Geometry: final body of the model. Coordinates: model frame, mm. Face numbers are marked on the shaded views. A direction names the side the tool comes from. Round coordinates to 2 decimals unless told otherwise and drop trailing zeros. Loops run counter-clockwise (first coordinate to the right, second up) from the corner with the lowest first, then second, coordinate; pieces in that order, holes last. Notation, with made-up numbers: (51, -18.75) - (67, -18.75) arc R19 cw to (67, 10.25) - close; hole circle Ø6 at (-22.75, 20). An arc over 180 degrees is marked (long way). Use CSV: the item, a comma, the result in double quotes.
from build123d import *

# Parameters (mm, degrees)
F1_DEPTH = 2
F3_DEPTH = 15
F4_R     = 3


with BuildPart() as f1:
    # F0 (on Top) → F1 (new body)
    with BuildSketch(Plane.XY):
        with BuildLine():
            ThreePointArc((46.9791666667, 17.11601295), (49.2390004637, 8.6902723394), (50, 0))
            ThreePointArc((50, 0), (49.2390004637, -8.6902723394), (46.9791666667, -17.11601295))
            ThreePointArc((46.9791666667, -17.11601295), (52.0440237461, -31.7330315504), (60, -45))
            ThreePointArc((60, -45), (67.9559762539, -31.7330315504), (73.0208333333, -17.11601295))
            ThreePointArc((73.0208333333, -17.11601295), (70, 0), (73.0208333333, 17.11601295))
            ThreePointArc((73.0208333333, 17.11601295), (67.9559762539, 31.7330315504), (60, 45))
            ThreePointArc((60, 45), (52.0440237461, 31.7330315504), (46.9791666667, 17.11601295))
        make_face()
        with BuildLine():
            ThreePointArc((46.9791666667, -17.11601295), (-50, 0), (46.9791666667, 17.11601295))
            ThreePointArc((46.9791666667, 17.11601295), (52.0440237461, 31.7330315504), (60, 45))
            ThreePointArc((60, 45), (-75, 0), (60, -45))
            ThreePointArc((60, -45), (52.0440237461, -31.7330315504), (46.9791666667, -17.11601295))
        make_face()
        with BuildLine():
            ThreePointArc((195, 0), (143.7170824513, 71.1512473538), (60, 45))
            ThreePointArc((60, 45), (67.9559762539, 31.7330315504), (73.0208333333, 17.11601295))
            ThreePointArc((73.0208333333, 17.11601295), (128.6902723394, 49.2390004637), (170, 0))
            ThreePointArc((170, 0), (128.6902723394, -49.2390004637), (73.0208333333, -17.11601295))
            ThreePointArc((73.0208333333, -17.11601295), (67.9559762539, -31.7330315504), (60, -45))
            ThreePointArc((60, -45), (143.7170824513, -71.1512473538), (195, 0))
        make_face()
        with BuildLine():
            ThreePointArc((46.9791666667, -17.11601295), (49.2390004637, -8.6902723394), (50, 0))
            ThreePointArc((50, 0), (49.2390004637, 8.6902723394), (46.9791666667, 17.11601295))
            ThreePointArc((46.9791666667, 17.11601295), (45, 0), (46.9791666667, -17.11601295))
        make_face()
        with BuildLine():
            ThreePointArc((75, 0), (74.5035653509, 8.6150304701), (73.0208333333, 17.11601295))
            ThreePointArc((73.0208333333, 17.11601295), (70, 0), (73.0208333333, -17.11601295))
            ThreePointArc((73.0208333333, -17.11601295), (74.5035653509, -8.6150304701), (75, 0))
        make_face()
    extrude(amount=F1_DEPTH)

    # F2 (on face) → F3 (join)
    with BuildSketch(Plane.XY.offset(2)):
        with BuildLine():
            ThreePointArc((60, 45), (-75, 0), (60, -45))
            ThreePointArc((60, -45), (195, 0), (60, 45))
        make_face()
        with BuildLine():
            ThreePointArc((60, -43.3128156554), (-74, 0), (60, 43.3128156554))
            ThreePointArc((60, 43.3128156554), (194, 0), (60, -43.3128156554))
        make_face(mode=Mode.SUBTRACT)
        with BuildLine():
            ThreePointArc((48.0208333333, -17.1755514023), (46, 0), (48.0208333333, 17.1755514023))
            ThreePointArc((48.0208333333, 17.1755514023), (-51, 0), (48.0208333333, -17.1755514023))
        make_face()
        with BuildLine():
            ThreePointArc((46.9791666667, -17.11601295), (-50, 0), (46.9791666667, 17.11601295))
            ThreePointArc((46.9791666667, 17.11601295), (45, 0), (46.9791666667, -17.11601295))
        make_face(mode=Mode.SUBTRACT)
        with BuildLine():
            ThreePointArc((71.9791666667, 17.1755514023), (74, 0), (71.9791666667, -17.1755514023))
            ThreePointArc((71.9791666667, -17.1755514023), (171, 0), (71.9791666667, 17.1755514023))
        make_face()
        with BuildLine():
            ThreePointArc((73.0208333333, 17.11601295), (170, 0), (73.0208333333, -17.11601295))
            ThreePointArc((73.0208333333, -17.11601295), (75, 0), (73.0208333333, 17.11601295))
        make_face(mode=Mode.SUBTRACT)
    extrude(amount=F3_DEPTH)

    # F4
    f4_edges = [f1.edges().sort_by_distance(p)[0] for p in [
        (60, 45, 8.5),
        (60, -45, 8.5),
        (60, 43.312816, 9.5),
        (71.979167, -17.175551, 9.5),
        (73.020833, -17.116013, 8.5),
        (73.020833, 17.116013, 8.5),
        (48.020833, 17.175551, 9.5),
        (46.979167, 17.116013, 8.5),
        (46.979167, -17.116013, 8.5),
        (60, -43.312816, 9.5),
        (48.020833, -17.175551, 9.5),
        (71.979167, 17.175551, 9.5),
    ]]
    fillet(f4_edges, radius=F4_R)


solid = f1.part
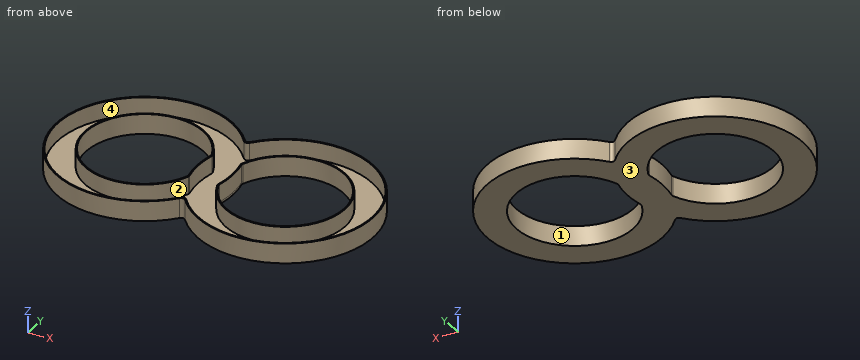
Item 1: Section C-C on z = 13. Give the number of separate pieces and of enclosed holes in the cut face, plus the area to 3 significant figures.
Final values:
separate pieces,"3"
enclosed holes,"3"
area,"1,380 mm²"
Item 2: Pin query (flat end, axial travel): P1, Ø3, axis at y = 26.5, z = 11.5, coming from the -X side; P2, Ø1.5, axis at x = -41.5, z = 5, coming from the -Y side; P3, Ø10, axis at x = -10, z = 7, coming from the -Y side. Return the tip coordinate at first contact, or that it passes through.
Final values:
P1,"stops at x = -70.71"
P2,"stops at y = -62.96"
P3,"stops at y = -74.83"
Item 3: Section B-B on y = 57.5. Return the cut outline in (x, z).
Final values:
outline,"(-48.15, 0) - (48.15, 0) - (48.15, 17) - (46.58, 17) - (46.58, 2) - (-46.58, 2) - (-46.58, 17) - (-48.15, 17) - close; (71.85, 0) - (168.15, 0) - (168.15, 17) - (166.58, 17) - (166.58, 2) - (73.42, 2) - (73.42, 17) - (71.85, 17) - close"
Item 4: Section D-D on y = -30. Return the cut outline in (x, z).
Final values:
outline,"(-68.74, 0) - (-40, 0) - (-40, 17) - (-41.24, 17) - (-41.24, 2) - (-67.65, 2) - (-67.65, 17) - (-68.74, 17) - close; (40, 0) - (80, 0) - (80, 17) - (78.76, 17) - (78.76, 2) - (41.24, 2) - (41.24, 17) - (40, 17) - close; (160, 0) - (188.74, 0) - (188.74, 17) - (187.65, 17) - (187.65, 2) - (161.24, 2) - (161.24, 17) - (160, 17) - close"
Item 5: Reachability of the marked faces 1 and 2 from +Z, -Z, +X, -X, +Y, -Y: full face, straight path, thin tool, end or side. Return the list, or none.
Final values:
face 1,"+Z, -Z"
face 2,"+Z"
Item 6: Section A-A on x = 120. Return the cut outline in (y, z), plus the area to 3 significant figures.
Final values:
outline,"(-75, 0) - (-50, 0) - (-50, 17) - (-51, 17) - (-51, 2) - (-74, 2) - (-74, 17) - (-75, 17) - close; (50, 0) - (75, 0) - (75, 17) - (74, 17) - (74, 2) - (51, 2) - (51, 17) - (50, 17) - close"
area,"160 mm²"
Item 7: Mould query, pull axis X, two halves, no side actions, for the marked faces 3 and 4. Classes: released by +X, released by -X, zero draft, split by the parting line, or undercut.
Final values:
face 3,"zero draft"
face 4,"undercut"
Item 8: Material intervals for line 1 (X direction, y = 0, z = 6.5); line 2 (Y direction, x = 0, z = 6.25); line 3 (X direction, y = -30.5, z = 6.5), sorted ascending.
Final values:
line 1,"x = -75 to -74, -51 to -50, 45 to 46, 74 to 75, 170 to 171, 194 to 195"
line 2,"y = -75 to -74, -51 to -50, 50 to 51, 74 to 75"
line 3,"x = -68.52 to -67.42, -40.87 to -39.62, 39.62 to 40.87, 79.13 to 80.38, 159.62 to 160.87, 187.42 to 188.52"
